Geometry: final body of the model. Coordinates: model frame, mm. Give positions to 0.01 mm unless a question says otherwise; leave off trailing zeros. Order: outer loops, then holes, each group sorted by start corner. A loop starts at its lowest first (then second) coordinate and runs counter-clockwise, first axis right, second up. Notation, with made-up numbers: (78, -20) -> (118, -20) arc R27 ccw to (118, -1) -> close; hole circle Ø8 at (77.25, 12.25). An arc over 180 degrees is marked (long way). Answer in a Markdown table with one row per item. Add a question column.
Q1. Cut plane B-B on y = 2. Return the cut outline in (x, z), and give its area (3 significant figures).
Q2. Contact query for flat-ended pins moving along their axis: P1, Ø8, axis at x = 7.5, y = -33.5, coming from the +Z side; P2, Ø4, axis at x = 13, z = -2.5, coming from the +Y side; P3, Ø5, axis at y = -23.5, z = -34.5, coming from the +X side. Output: stop coordinate, or through.
Q3. Cut plane A-A on x = -5.5. Return the cut outline in (y, z), and give its area (3 significant figures).
Q4. Line query: line 1 along Z through (x, y) = (40, 41.5); line 2 along X through (y, z) = (12, 46.5); line 3 along X through (y, z) = (6, 30). Output: solid intervals per line, ascending. Write a range as from..to.
from build123d import *

# Parameters (mm, degrees)
F_10_0_10_DURCHMESSER_BOHRUNG1_D                     = 10
F_10_0_10_DURCHMESSER_BOHRUNG1_DEPTH                 = 22.64
F_10_0_10_DURCHMESSER_BOHRUNG1_CSINK_D               = 10.05
F_10_0_10_DURCHMESSER_BOHRUNG1_CSINK_ANGLE           = 90
F_10_0_10_DURCHMESSER_BOHRUNG1_TIP                   = 3.004303095
F_10_0_10_DURCHMESSER_BOHRUNG1_ON_FACE_2_D           = 10
F_10_0_10_DURCHMESSER_BOHRUNG1_ON_FACE_2_DEPTH       = 22.64
F_10_0_10_DURCHMESSER_BOHRUNG1_ON_FACE_2_CSINK_D     = 10.05
F_10_0_10_DURCHMESSER_BOHRUNG1_ON_FACE_2_CSINK_ANGLE = 90
F_10_0_10_DURCHMESSER_BOHRUNG1_ON_FACE_2_TIP         = 3.004303095
F_10_0_10_DURCHMESSER_BOHRUNG1_ON_FACE_3_D           = 10
F_10_0_10_DURCHMESSER_BOHRUNG1_ON_FACE_3_DEPTH       = 22.64
F_10_0_10_DURCHMESSER_BOHRUNG1_ON_FACE_3_CSINK_D     = 10.05
F_10_0_10_DURCHMESSER_BOHRUNG1_ON_FACE_3_CSINK_ANGLE = 90
F_10_0_10_DURCHMESSER_BOHRUNG1_ON_FACE_3_TIP         = 3.004303095


with BuildPart() as part:
    # Skizze1 → Rotation1 (revolve)
    with BuildSketch(Plane.XY):
        with BuildLine():
            Line((0, 60), (0, -60))
            ThreePointArc((0, -60), (60, 0), (0, 60))
        make_face()
    revolve(axis=Axis((0, 60, 0), (0, -1, 0)))

    # 10.0 _10_ Durchmesser Bohrung1
    with Locations(Plane(origin=(38.060989939, 46.377923621, 0.670257752), x_dir=(0.773013628, -0.634389416, 0), z_dir=(0.634349832, 0.772965394, 0.011170963))):
        with Locations((0, 0)):
            CounterSinkHole(F_10_0_10_DURCHMESSER_BOHRUNG1_D / 2, F_10_0_10_DURCHMESSER_BOHRUNG1_CSINK_D / 2, depth=F_10_0_10_DURCHMESSER_BOHRUNG1_DEPTH, counter_sink_angle=F_10_0_10_DURCHMESSER_BOHRUNG1_CSINK_ANGLE)
            with Locations((0, 0, -(F_10_0_10_DURCHMESSER_BOHRUNG1_DEPTH + F_10_0_10_DURCHMESSER_BOHRUNG1_TIP / 2))):  # 118° drill point
                Cone(0, F_10_0_10_DURCHMESSER_BOHRUNG1_D / 2, F_10_0_10_DURCHMESSER_BOHRUNG1_TIP, mode=Mode.SUBTRACT)

    # 10.0 _10_ Durchmesser Bohrung1 on face 2
    with Locations(Plane(origin=(-21.137326584, 56.151455854, 0.476896544), x_dir=(0.935887137, 0.352299968, 0), z_dir=(-0.35228884, 0.935857576, 0.007947996))):
        with Locations((0, 0)):
            CounterSinkHole(F_10_0_10_DURCHMESSER_BOHRUNG1_ON_FACE_2_D / 2, F_10_0_10_DURCHMESSER_BOHRUNG1_ON_FACE_2_CSINK_D / 2, depth=F_10_0_10_DURCHMESSER_BOHRUNG1_ON_FACE_2_DEPTH, counter_sink_angle=F_10_0_10_DURCHMESSER_BOHRUNG1_ON_FACE_2_CSINK_ANGLE)
            with Locations((0, 0, -(F_10_0_10_DURCHMESSER_BOHRUNG1_ON_FACE_2_DEPTH + F_10_0_10_DURCHMESSER_BOHRUNG1_ON_FACE_2_TIP / 2))):  # 118° drill point
                Cone(0, F_10_0_10_DURCHMESSER_BOHRUNG1_ON_FACE_2_D / 2, F_10_0_10_DURCHMESSER_BOHRUNG1_ON_FACE_2_TIP, mode=Mode.SUBTRACT)

    # 10.0 _10_ Durchmesser Bohrung1 on face 3
    with Locations(Plane(origin=(5.885070461, 34.684297812, -48.604170922), x_dir=(0, -0.813994513, -0.580872562), z_dir=(0.098084936, 0.578071622, -0.81006947))):
        with Locations((0, 0)):
            CounterSinkHole(F_10_0_10_DURCHMESSER_BOHRUNG1_ON_FACE_3_D / 2, F_10_0_10_DURCHMESSER_BOHRUNG1_ON_FACE_3_CSINK_D / 2, depth=F_10_0_10_DURCHMESSER_BOHRUNG1_ON_FACE_3_DEPTH, counter_sink_angle=F_10_0_10_DURCHMESSER_BOHRUNG1_ON_FACE_3_CSINK_ANGLE)
            with Locations((0, 0, -(F_10_0_10_DURCHMESSER_BOHRUNG1_ON_FACE_3_DEPTH + F_10_0_10_DURCHMESSER_BOHRUNG1_ON_FACE_3_TIP / 2))):  # 118° drill point
                Cone(0, F_10_0_10_DURCHMESSER_BOHRUNG1_ON_FACE_3_D / 2, F_10_0_10_DURCHMESSER_BOHRUNG1_ON_FACE_3_TIP, mode=Mode.SUBTRACT)


solid = part.part
Completed:
| question | item | result |
|---|---|---|
| 1 | outline | circle Ø119.93 at (0, 0) |
| 1 | area | 11,300 mm² |
| 2 | P1 | stops at z = 51.77 |
| 2 | P2 | stops at y = 58.94 |
| 2 | P3 | stops at x = 45.39 |
| 3 | outline | circle Ø119.49 at (0, 0) |
| 3 | area | 11,200 mm² |
| 4 | line 1 | z = -16.67..-1.33, 2.62..16.67 |
| 4 | line 2 | x = -35.97..35.97 |
| 4 | line 3 | x = -51.61..51.61 |
